Part model, mm, in its own coordinate system. A direction names the side the tool comes from. Round coordinates to 2 decimals unless told otherwise and drop trailing zeros. Write each loop counter-clockwise with the first axis right and the second up, starting at its lowest first coordinate (ties: lowest second). Pieces come first, ordered by that corner, then holes.
```python
from build123d import *

# Parameters (mm, degrees)
SKETCH1_W                        = 31.75
SKETCH1_H                        = 31.75
STOCK_DEPTH                      = 50.8
SP_TAP_D                         = 12.7
SP_TAP_DEPTH                     = 33.02
SP_TAP_TIP                       = 3.815464931
F_47_START                       = -7.737817178
F_47_0_0785_GOX_ORFICE_OUTLINE_R = 0.99695
F_47_0_0785_GOX_ORFICE_DEPTH     = 11.439445718
F_65_0_035_DIAMETER_HOLE2_REACH  = 63.974
F_65_0_035_DIAMETER_HOLE2_BORE_R = 0.4445
SKETCH25_W                       = 31.75
SKETCH25_H                       = 31.75
BOSS_EXTRUDE1_DEPTH              = 6.35
M14_TAPPED_HOLE1_D               = 12
M14_TAPPED_HOLE1_DEPTH           = 19.05
M14_TAPPED_HOLE1_CSINK_D         = 14.05
M14_TAPPED_HOLE1_CSINK_ANGLE     = 90
M14_TAPPED_HOLE1_TIP             = 3.605163714
SKETCH30_R                       = 6.0198
CUT_EXTRUDE1_DEPTH               = 62.401577893
SKETCH31_R                       = 25.0825
SKETCH31_R_2                     = 1.5875
SKETCH31_W                       = 31.75
SKETCH31_H                       = 31.75
BOSS_EXTRUDE2_DEPTH              = 6.35
F_1_4_0_25_DIAMETER_HOLE1_D      = 6.35
F_1_4_0_25_DIAMETER_HOLE1_DEPTH  = 3.175
F_1_4_0_25_DIAMETER_HOLE1_TIP    = 1.907732465
FILLET2_R                        = 6.35
FILLET3_R                        = 6.35
FILLET4_R                        = 1.5875


# Read off the part's stored shape, not the designer's step: #47 (0.0785) GOx Orfice
with BuildPart() as part:
    # Sketch1 → Stock (new body)
    with BuildSketch(Plane(origin=(0, 0, 0), x_dir=(1, 0, 0), z_dir=(0, 1, 0))):
        Rectangle(SKETCH1_W, SKETCH1_H)
    extrude(amount=STOCK_DEPTH)

    # SP TAP
    with Locations(Plane(origin=(0, 50.8, 0), x_dir=(1, 0, 0), z_dir=(0, 1, 0))):
        with Locations((0, 0)):
            Hole(SP_TAP_D / 2, depth=SP_TAP_DEPTH)
            with Locations((0, 0, -(SP_TAP_DEPTH + SP_TAP_TIP / 2))):  # 118° drill point
                Cone(0, SP_TAP_D / 2, SP_TAP_TIP, mode=Mode.SUBTRACT)

    # #47 (0.0785) GOx Orfice outline → #47 (0.0785) GOx Orfice (cut)
    with BuildSketch(Plane(origin=(0, 0, 0), x_dir=(1, 0, 0), z_dir=(0, 0.42261826174069705, 0.9063077870366512)).offset(F_47_START)):
        with Locations((0, 21.96659786)):
            Circle(F_47_0_0785_GOX_ORFICE_OUTLINE_R)
    f_47_0_0785_gox_orfice = extrude(amount=F_47_0_0785_GOX_ORFICE_DEPTH, mode=Mode.SUBTRACT)

    # Second GOx Orfice: #47 (0.0785) GOx Orfice across plane
    add(f_47_0_0785_gox_orfice.mirror(Plane.XY), mode=Mode.SUBTRACT)

    # #65 (0.035) Diameter Hole2 bore → #65 (0.035) Diameter Hole2 (cut, up to next)
    with BuildSketch(Plane(origin=(15.875, 0, 0), x_dir=(0, 0, -1), z_dir=(1, 0, 0)), mode=Mode.PRIVATE) as f_65_0_035_diameter_hole2_sk1:
        with Locations((5.715, 25.4)):
            Circle(F_65_0_035_DIAMETER_HOLE2_BORE_R)
    f_65_0_035_diameter_hole2_tool1 = extrude(f_65_0_035_diameter_hole2_sk1.sketch, amount=-F_65_0_035_DIAMETER_HOLE2_REACH, mode=Mode.PRIVATE) & part.part
    add(f_65_0_035_diameter_hole2_tool1.solids().sort_by_distance((15.875, 25.4, -5.715))[0], mode=Mode.SUBTRACT)

    # Sketch25 → Boss-Extrude1 (add)
    with BuildSketch(Plane(origin=(0, 0, 0), x_dir=(-1, 0, 0), z_dir=(0, -1, 0))):
        Rectangle(SKETCH25_W, SKETCH25_H)
    extrude(amount=BOSS_EXTRUDE1_DEPTH)

    # M14 Tapped Hole1
    with Locations(Plane(origin=(0, -6.35, 0), x_dir=(-1, 0, 0), z_dir=(0, -1, 0))):
        with Locations((0, 0)):
            CounterSinkHole(M14_TAPPED_HOLE1_D / 2, M14_TAPPED_HOLE1_CSINK_D / 2, depth=M14_TAPPED_HOLE1_DEPTH, counter_sink_angle=M14_TAPPED_HOLE1_CSINK_ANGLE)
            with Locations((0, 0, -(M14_TAPPED_HOLE1_DEPTH + M14_TAPPED_HOLE1_TIP / 2))):  # 118° drill point
                Cone(0, M14_TAPPED_HOLE1_D / 2, M14_TAPPED_HOLE1_TIP, mode=Mode.SUBTRACT)

    # Sketch30 → Cut-Extrude1 (cut, through all)
    with BuildSketch(Plane(origin=(0, -6.35, 0), x_dir=(-1, 0, 0), z_dir=(0, -1, 0))):
        with Locations(Location((0, 0, 0), (0, 0, 90))):
            Circle(SKETCH30_R)
    extrude(amount=-CUT_EXTRUDE1_DEPTH, mode=Mode.SUBTRACT)

    # Sketch31 → Boss-Extrude2 (add)
    with BuildSketch(Plane(origin=(0, 50.8, 0), x_dir=(1, 0, 0), z_dir=(0, 1, 0))):
        with Locations(Location((0, 0, 0), (0, 0, 270))):
            Circle(SKETCH31_R)
        with Locations(Location((21.2725, 0, 0), (0, 0, 270))):
            Circle(SKETCH31_R_2, mode=Mode.SUBTRACT)
        with Locations(Location((0, -21.2725, 0), (0, 0, 270))):
            Circle(SKETCH31_R_2, mode=Mode.SUBTRACT)
        with Locations(Location((-21.2725, 0, 0), (0, 0, 270))):
            Circle(SKETCH31_R_2, mode=Mode.SUBTRACT)
        with Locations(Location((0, 21.2725, 0), (0, 0, 270))):
            Circle(SKETCH31_R_2, mode=Mode.SUBTRACT)
        Rectangle(SKETCH31_W, SKETCH31_H, mode=Mode.SUBTRACT)
    extrude(amount=-BOSS_EXTRUDE2_DEPTH)

    # 1/4 (0.25) Diameter Hole1
    with Locations(Plane(origin=(15.875, 0, 0), x_dir=(0, 0, -1), z_dir=(1, 0, 0))):
        with Locations((5.715, 25.4)):
            Hole(F_1_4_0_25_DIAMETER_HOLE1_D / 2, depth=F_1_4_0_25_DIAMETER_HOLE1_DEPTH)
            with Locations((0, 0, -(F_1_4_0_25_DIAMETER_HOLE1_DEPTH + F_1_4_0_25_DIAMETER_HOLE1_TIP / 2))):  # 118° drill point
                Cone(0, F_1_4_0_25_DIAMETER_HOLE1_D / 2, F_1_4_0_25_DIAMETER_HOLE1_TIP, mode=Mode.SUBTRACT)

    # Sketch35 → Cut-Revolve1 (revolve, cut)
    with BuildSketch(Plane(origin=(0, 0, 0), x_dir=(0, 0, -1), z_dir=(1, 0, 0)), mode=Mode.PRIVATE) as cut_revolve1_sk:
        Polygon((11.1125, 19.055615182), (11.499679808, 15.37184538), (19.76016519, 11.519917786), (21.101978171, 14.39744501), (15.875, 16.83482496), align=None)
    cut_revolve1 = revolve(cut_revolve1_sk.sketch.rotate(Axis((0, 16.83482496, -15.875), (0, 0.4226182617406968, 0.9063077870366512)), 180), axis=Axis((0, 16.83482496, -15.875), (0, 0.4226182617406968, 0.9063077870366512)), mode=Mode.SUBTRACT)

    # Mirror1: Cut-Revolve1 across plane
    add(cut_revolve1.mirror(Plane.XY), mode=Mode.SUBTRACT)

    # Fillet2
    fillet2_edges = [part.edges().sort_by_distance(p)[0] for p in [
        (-15.875, 19.05, 15.875),
        (15.875, 19.05, 15.875),
        (-15.875, 19.05, -15.875),
        (15.875, 19.05, -15.875),
    ]]
    fillet(fillet2_edges, radius=FILLET2_R)

    # Fillet3
    fillet3_edges = [part.edges().sort_by_distance(p)[0] for p in [
        (0, -6.35, 15.875),
        (15.875, -6.35, 0),
        (-15.875, -6.35, 0),
        (0, -6.35, -15.875),
        (-14.015128061, -6.35, -14.015128061),
        (14.015128061, -6.35, -14.015128061),
        (14.015128061, -6.35, 14.015128061),
        (-14.015128061, -6.35, 14.015128061),
    ]]
    fillet(fillet3_edges, radius=FILLET3_R)

    # Fillet4
    fillet4_edges = [part.edges().sort_by_distance(p)[0] for p in [
        (0, 44.45, 15.875),
        (-15.875, 44.45, 0),
        (15.875, 44.45, 0),
        (0, 44.45, -15.875),
        (-14.015128061, 44.45, 14.015128061),
        (14.015128061, 44.45, 14.015128061),
        (14.015128061, 44.45, -14.015128061),
        (-14.015128061, 44.45, -14.015128061),
    ]]
    fillet(fillet4_edges, radius=FILLET4_R)


solid = part.part
```
Q1. Which spindle directions (+Z, -Z, +X, -X, +Y, -Y) get a long thin tool onto all of the face, cutting with end or side? Do faces 4 (the flat face through (0, 22, -15.875)), 5 (the cylindrical face through (13.97, 21.13, 14.06)), 6 (the flat face through (19, 44.45, 2)), 7 (the flat face through (15.875, 22, 0)). Say none if no direction does.
Values follow:
face 4: -Z, +X, -X, -Y
face 5: +Z, +X, -Y
face 6: -Y
face 7: +Z, -Z, +X, -Y
Q2. Drop flat-ended pins along their axis: pin 1 (8.5 mm diameter, centred on y = 25.4, z = -5.715, fed in from -X) (3 decimals); pin 2 (2.5 mm diameter, centred on x = 0, z = -21.27, fed in from +Y); pin 3 (15 mm diameter, centred on x = 3.5, y = 13.5, fed in from +Z) (3 decimals); pin 4 (6 mm diameter, centred on x = 4, y = 28.5, fed in from -Z) (3 decimals). Give the stop position or say it passes through.
Values follow:
pin 1: stops at x = -15.875
pin 2: passes through
pin 3: stops at z = 15.875
pin 4: stops at z = -15.875
Q3. Wall check: L1, parallel to Z at x = 0, y = 4.75 (3 decimals); L2, parallel to Y at x = 17, z = -14.5; L3, parallel to Z at x = 0, y = 39 (3 decimals). Give the ranges that are in metal, low to high.
Values follow:
L1: z = -15.875 to -6.02, 6.02 to 15.875
L2: y = 44.45 to 50.8
L3: z = -15.875 to -6.35, 6.35 to 15.875
Q4. Cut at B-B on z = 0. State how many separate pieces and enclosed holes the cut face has, plus the area to 3 significant figures.
Values follow:
separate pieces: 4
enclosed holes: 0
area: 1,160 mm2
Q5. Cut at A-A on y = 41. Write the cut outline in (x, z) (3 decimals).
Values follow:
outline: (-15.875, -9.525) arc R6.35 ccw to (-9.525, -15.875) - (9.525, -15.875) arc R6.35 ccw to (15.875, -9.525) - (15.875, 9.525) arc R6.35 ccw to (9.525, 15.875) - (-9.525, 15.875) arc R6.35 ccw to (-15.875, 9.525) - close; hole circle Ø12.7 at (0, 0)
Q6. Mould opens along X. For faces 1 (the cylindrical face through (14.265, 28.548, -6.128)), 2 (the cylindrical face through (-0.14, 14.544, 13.283)), 3 (the cylindrical face through (-13.97, 21.73, -14.06)) say: +X half, -X half, draft (parallel to the pull), parting line (faces both ways), or undercut.
Values follow:
face 1: draft
face 2: undercut
face 3: -X half
